For this review, take the finished solid that the model builds, in its own axes (mm). A direction names the side the tool comes from. Give positions to 0.01 mm unless a question says otherwise; leave off trailing zeros. Write each loop counter-clockwise with the first axis right and the second up, starting at its lowest first coordinate (ties: lowest second). Pieces come first, ordered by that corner, then holes. Notation, with made-up numbers: (67, 49.5) -> (83, 49.5) arc R28 cw to (83, 68.5) -> close; hole circle Ø5 at (-22.5, 41.5). An arc over 180 degrees is marked (long way). Return JSON: item names as keys, results as strings.
from build123d import *

# Parameters (mm, degrees)
BOSS_EXTRUDE1_DEPTH = 3
CUT_EXTRUDE1_DEPTH  = 4
FILLET1_R           = 5
SKETCH3_W           = 3
SKETCH3_H           = 5
BOSS_EXTRUDE2_DEPTH = 3


with BuildPart() as part:
    # Sketch1 → Boss-Extrude1 (new body)
    with BuildSketch(Plane(origin=(0, 0, 0), x_dir=(0, 0, -1), z_dir=(1, 0, 0))):
        with BuildLine():
            Line((-13.75, 11.75), (-30, 11.75))
            Line((-30, 11.75), (-30, -11.75))
            Line((-30, -11.75), (30, -11.75))
            Line((30, -11.75), (30, 11.75))
            Line((30, 11.75), (13.75, 11.75))
            ThreePointArc((13.75, 11.75), (0, -2), (-13.75, 11.75))
        make_face()
    extrude(amount=BOSS_EXTRUDE1_DEPTH)

    # Sketch2 → Cut-Extrude1 (cut, through all)
    with BuildSketch(Plane(origin=(3, 0, 0), x_dir=(0, 0, -1), z_dir=(1, 0, 0))):
        with BuildLine():
            Line((-25, 6.25), (-30, 6.25))
            Line((-30, 6.25), (-30, 3.25))
            Line((-30, 3.25), (-25, 3.25))
            ThreePointArc((-25, 3.25), (-23.5, 4.75), (-25, 6.25))
        make_face()
    cut_extrude1 = extrude(amount=-CUT_EXTRUDE1_DEPTH, mode=Mode.SUBTRACT)

    # Mirror2: Cut-Extrude1 across plane
    add(cut_extrude1.mirror(Plane.XY), mode=Mode.SUBTRACT)

    # Fillet1
    fillet1_edges = [part.edges().sort_by_distance(p)[0] for p in [
        (1.5, 11.75, 30),
        (1.5, 11.75, -30),
    ]]
    fillet(fillet1_edges, radius=FILLET1_R)

    # Sketch3 → Boss-Extrude2 (add)
    with BuildSketch(Plane.XZ.offset(11.75)):
        with Locations((1.5, 17.5)):
            Rectangle(SKETCH3_W, SKETCH3_H)
    boss_extrude2 = extrude(amount=BOSS_EXTRUDE2_DEPTH)

    # Mirror3: Boss-Extrude2 across plane
    add(boss_extrude2.mirror(Plane.XY))


solid = part.part
1. The part is to be moulded in two halves that separate along Z. For faces 4 (the flat face through (1, -4, -30)), 5 (the flat face through (1, -11.75, 25)), 6 (the cylindrical face through (1, -2, 0)), 7 (the flat face through (1, -13, -15)), say which applies: +Z half, -Z half, draft (parallel to the pull), parting line (faces both ways), or undercut.
Results found:
{"face 4": "-Z half", "face 5": "draft", "face 6": "undercut", "face 7": "undercut"}
2. Add section D-D, the plane z = 9.5. State the section outline as (x, y) points.
Results found:
{"outline": "(0, -11.75) -> (3, -11.75) -> (3, 1.81) -> (0, 1.81) -> close"}
3. For pin 1 (1.5 mm diameter, centred on x = 1.5, z = -1.5, fed in from -Y); pin 2 (1.5 mm diameter, centred on x = 0.5, z = -1, fed in from +Y); pin 3 (0.9 mm diameter, centred on x = 1.5, y = -13.5, fed in from +Z), all flat-tipped, find the tip position at first contact; note any pin that passes through.
Results found:
{"pin 1": "stops at y = -11.75", "pin 2": "stops at y = -1.89", "pin 3": "stops at z = 20"}
4. To check wall thickness, follow probe 1 along Z at (x, y) = (1.4, -12.75); probe 2 along Y at (x, z) = (2.5, -20.5); probe 3 along Y at (x, z) = (1.9, 27). State the ranges of each line that lie inside material, in increasing order.
Results found:
{"probe 1": "z = -20 to -15, 15 to 20", "probe 2": "y = -11.75 to 11.75", "probe 3": "y = -11.75 to 3.25, 6.25 to 11.33"}
5. Add section B-B, the plane x = 0.8. State the section outline as (y, z) points, plus the area to 3 significant figures.
Results found:
{"outline": "(-14.75, -20) -> (-11.75, -20) -> (-11.75, -30) -> (3.25, -30) -> (3.25, -25) arc R1.5 cw to (6.25, -25) -> (6.25, -30) -> (6.75, -30) arc R5 ccw to (11.75, -25) -> (11.75, -13.75) arc R13.75 cw to (11.75, 13.75) -> (11.75, 25) arc R5 ccw to (6.75, 30) -> (6.25, 30) -> (6.25, 25) arc R1.5 cw to (3.25, 25) -> (3.25, 30) -> (-11.75, 30) -> (-11.75, 20) -> (-14.75, 20) -> (-14.75, 15) -> (-11.75, 15) -> (-11.75, -15) -> (-14.75, -15) -> close", "area": "1,100 mm²"}
6. Add section A-A, the plane y = 4.75. State the section outline as (x, z) points.
Results found:
{"outline": "(0, -23.5) -> (3, -23.5) -> (3, -11.83) -> (0, -11.83) -> close; (0, 11.83) -> (3, 11.83) -> (3, 23.5) -> (0, 23.5) -> close"}
7. For faces 1 (the flat face through (1, -11.75, 0)), 2 (the flat face through (1, -13, 20)), 3 (the flat face through (2, 3.25, -28)), list the 3-axis set-ups (+Z, -Z, +X, -X, +Y, -Y) from which the entire face can be reached by the end or side of a thin tool; tool diameter is ignored.
Results found:
{"face 1": "+X, -X, -Y", "face 2": "+Z, +X, -X, -Y", "face 3": "-Z, +X, -X"}
8. Add section C-C, the plane z = 0. State the section outline as (x, y) points.
Results found:
{"outline": "(0, -11.75) -> (3, -11.75) -> (3, -2) -> (0, -2) -> close"}
